Design review of the part built by this model. Coordinates are the model's own, in mm. A direction names the side the tool comes from. Coordinates: 2 decimals unless noted, no trailing zeros. Loops run counter-clockwise (first coordinate to the right, second up) from the corner with the lowest first, then second, coordinate; pieces in that order, holes last. Notation, with made-up numbers: (13.25, -28.5) -> (41.25, -28.5) arc R19 cw to (41.25, -12.5) -> close; hole circle Ø7 at (-37.5, 48.5). An arc over 180 degrees is marked (long way). Use a Markdown table: item, result. Add a question column.
Q1. Take a section at D-D on y = -13. Write out the cut boundary in (x, z), plus the area to 3 significant figures.
Q2. Take a section at C-C on y = -39. Write out the cut boundary in (x, z).
Q3. For faces 4 (the face through (-4, 1, 0)), 5 (the face through (-24, 39, 3)), 6 (the face through (13.338, -32.494, 3.549)), list the 3-axis set-ups (+Z, -Z, +X, -X, +Y, -Y) from which the entire face can be reached by the end or side of a thin tool; tool diameter is ignored.
Q4. Take a section at B-B on z = 3.25. Write out the cut boundary in (x, y) (3 decimals), plus the area to 3 significant figures.
Q5. Draft analysis for pull direction Y (two halves, no side actions). For faces 1 (the face through (-16.068, -5.044, 3.549)), 2 (the face through (-22.5, -16, 3)), 3 (the face through (-15, 45, 3)), state which applies: pulls with the +Y half, pulls with the -Y half, needs draft (parallel to the pull), parting line crosses it, or undercut.
Q6. Clearance check with flat-ended pins moving along their axes: pin 1 Ø3.5 at (x, z) = (-28.5, 5) entering from -Y; pin 2 Ø3.5 at (y, z) = (33, 2.5) entering from -X; pin 3 Ø2 at (x, z) = (-15, 5) entering from -Y. State where each tip first meets the part, or that it passes through.
Q7. For probe 1 along X at (y, z) = (-7, 2.25); probe 2 along X at (y, z) = (-5, 2.25); probe 3 along Y at (x, z) = (-23, 2), list the stretches that pass through material, from the lowest coordinate up.
Q8. Take a section at A-A on x = -20. Write out the cut boundary in (y, z), plus the area to 3 significant figures.
from build123d import *

# Parameters (mm, degrees)
F1_DEPTH = 7
F2_D     = 2
F3_D     = 5.75
F4_DEPTH = 16
F5_DEPTH = 5


with BuildPart() as f1:
    # F0 (on Top) → F1 (new body)
    with BuildSketch(Plane.XY):
        Polygon((10.5, -45), (22.5, -45), (22.5, 17.153987661), (0, 45), (-14.5, 45), (-14.5, 39), (-22.5, 39), (-22.5, 16), (-14.5, 16), (-14.5, 10), (-22.5, 10), (-22.5, -42.25), (-10.5080957781, -42.25), (-10.6281967604, -1.0001864958), (10.3717142302, -0.9390441602), align=None)
    extrude(amount=F1_DEPTH)

    # F2 (through all)
    with Locations(Plane(origin=(0, 0, 0), x_dir=(1, 0, 0), z_dir=(0, 0, -1))):
        with Locations((-17.0669870824, 5), (-17.7734121563, 37), (17.7265878437, 39), (17.9330129176, 7)):
            Hole(F2_D / 2)

    # F3 (through all)
    with Locations(Plane(origin=(0, 0, 0), x_dir=(1, 0, 0), z_dir=(0, 0, -1))):
        with Locations((-10.5364832571, 32.5000529818), (10.4634277335, 32.4389106462)):
            Hole(F3_D / 2)

    # F4 (add): faces of the model
    f4_faces = [f1.faces().sort_by_distance(p)[0] for p in [
        (-14.5, 42, 3.5),
        (-14.5, 13, 3.5),
    ]]
    extrude(f4_faces, amount=F4_DEPTH)

    # F5 (cut): a face of the model
    f5_faces = [f1.faces().sort_by_distance(p)[0] for p in [
        (-22.5, 27.5, 3.5),
    ]]
    extrude(f5_faces, amount=-F5_DEPTH, mode=Mode.SUBTRACT)


solid = f1.part
Answer list:
| question | item | result |
|---|---|---|
| 1 | outline | (-22.5, 0) -> (-10.59, 0) -> (-10.59, 7) -> (-22.5, 7) -> close; (10.41, 0) -> (22.5, 0) -> (22.5, 7) -> (10.41, 7) -> close |
| 1 | area | 168 mm² |
| 2 | outline | (-22.5, 0) -> (-10.52, 0) -> (-10.52, 7) -> (-22.5, 7) -> close; (10.48, 0) -> (16.73, 0) -> (16.73, 7) -> (10.48, 7) -> close; (18.73, 0) -> (22.5, 0) -> (22.5, 7) -> (18.73, 7) -> close |
| 3 | face 4 | -Z, +X, -X, +Y, -Y |
| 3 | face 5 | +Z, -Z, -X |
| 3 | face 6 | +Z, -Z |
| 4 | outline | (-30.5, 10) -> (-22.5, 10) -> (-22.5, -42.25) -> (-10.508, -42.25) -> (-10.528, -35.375) arc R2.875 cw to (-10.545, -29.625) -> (-10.628, -1) -> (10.372, -0.939) -> (10.455, -29.564) arc R2.875 cw to (10.472, -35.314) -> (10.5, -45) -> (22.5, -45) -> (22.5, 17.154) -> (0, 45) -> (-30.5, 45) -> (-30.5, 39) -> (-17.5, 39) -> (-17.5, 16) -> (-30.5, 16) -> close; hole circle Ø2 at (-17.773, -37); hole circle Ø2 at (-17.067, -5); hole circle Ø2 at (17.727, -39); hole circle Ø2 at (17.933, -7) |
| 4 | area | 2,720 mm² |
| 5 | face 1 | undercut |
| 5 | face 2 | needs draft |
| 5 | face 3 | pulls with the +Y half |
| 6 | pin 1 | y = 10 |
| 6 | pin 2 | x = -17.5 |
| 6 | pin 3 | y = -42.25 |
| 7 | probe 1 | -22.5 to -10.61, 10.39 to 16.93, 18.93 to 22.5 |
| 7 | probe 2 | -22.5 to -18.07, -16.07 to -10.62, 10.38 to 22.5 |
| 7 | probe 3 | 10 to 16, 39 to 45 |
| 8 | outline | (-42.25, 0) -> (16, 0) -> (16, 7) -> (-42.25, 7) -> close; (39, 0) -> (45, 0) -> (45, 7) -> (39, 7) -> close |
| 8 | area | 450 mm² |
